Part model, mm, in its own coordinate system. A direction names the side the tool comes from. Give positions to 0.01 mm unless a question says otherwise; leave off trailing zeros. Order: outer loops, then holes, each group sorted by start corner. A loop starts at its lowest first (then second) coordinate and runs counter-clockwise, first axis right, second up. Notation, with made-up numbers: (52.25, 6.5) -> (110.25, 6.5) arc R22 cw to (110.25, 28.5) -> close; hole circle Ø8 at (61, 8). An arc over 180 degrees is marked (long way). Write item = value, one per line. Start each with the question number.
(1) Which spindle directions (+Z, -Z, +X, -X, +Y, -Y) get a long thin tool onto all of the face, cutting with end or side? Do faces 1 (the flat face through (2, 25, 3)), 2 (the flat face through (-21, 10, 3)), 3 (the flat face through (-21, 25, 3)), 4 (the flat face through (0, 0, 2)). Say none if no direction does.
(2) Saw through at C-C, the plane y = 3.5. List the corners of the cut face in (x, z), then the cut area to 3 significant figures.
(3) Saw through at A-A, the plane z = 0.75. List the corners of the cut face in (x, y).
(4) Saw through at D-D, the plane x = -20.5. List the corners of the cut face in (y, z).
(5) Probe line 1 along Y through (x, z) = (-20.5, 4.05); line 2 along Y through (x, z) = (2.5, 3.4); line 3 along Y through (x, z) = (-14, 2.55). List the from-to ranges inside material, lowest first. Write a range as from..to.
(6) Flat gauge pins, fed straight in: pin 1 (2.5 mm diameter, centred on y = 23.5, z = 1.5, fed in from -X); pin 2 (2.5 mm diameter, centred on x = -5.5, z = 3, fed in from +Y); pin 3 (1.5 mm diameter, centred on x = -13.5, z = 3, fed in from -Y); pin 4 (4 mm diameter, centred on x = 2.5, y = 31.5, fed in from +Z). Where does each tip first touch, or does it go through?
(7) Saw through at B-B, the plane x = 2.5. List the corners of the cut face in (y, z).
from build123d import *

# Parameters (mm, degrees)
SKETCH1_W           = 18
SKETCH1_H           = 35
BOSS_EXTRUDE1_DEPTH = 5
SKETCH2_W           = 5
SKETCH2_H           = 20
BOSS_EXTRUDE2_DEPTH = 5
SKETCH3_W           = 9
SKETCH3_H           = 5
BOSS_EXTRUDE3_DEPTH = 5
SKETCH4_W           = 5
SKETCH4_H           = 15
BOSS_EXTRUDE4_DEPTH = 5
SKETCH5_W           = 9
SKETCH5_H           = 5
BOSS_EXTRUDE5_DEPTH = 5
SKETCH6_R           = 2.1
CUT_EXTRUDE1_DEPTH  = 5
BOSS_EXTRUDE6_DEPTH = 5
SKETCH8_R           = 2.1
CUT_EXTRUDE2_DEPTH  = 5
BOSS_EXTRUDE7_DEPTH = 5


with BuildPart() as part:
    # Sketch1 → Boss-Extrude1 (new body)
    with BuildSketch(Plane.XY):
        with Locations((-9, 17.5)):
            Rectangle(SKETCH1_W, SKETCH1_H)
    extrude(amount=BOSS_EXTRUDE1_DEPTH)

    # Sketch2 → Boss-Extrude2 (add)
    with BuildSketch(Plane(origin=(0, 0, 0), x_dir=(0, 0, -1), z_dir=(1, 0, 0))):
        with Locations((-2.5, 15)):
            Rectangle(SKETCH2_W, SKETCH2_H)
    extrude(amount=BOSS_EXTRUDE2_DEPTH)

    # Sketch3 → Boss-Extrude3 (add)
    with BuildSketch(Plane.XZ):
        with Locations((-4.5, 2.5)):
            Rectangle(SKETCH3_W, SKETCH3_H)
    extrude(amount=BOSS_EXTRUDE3_DEPTH)

    # Sketch4 → Boss-Extrude4 (add)
    with BuildSketch(Plane.XY.offset(5)):
        with Locations((-20.5, 17.5)):
            Rectangle(SKETCH4_W, SKETCH4_H)
    extrude(amount=-BOSS_EXTRUDE4_DEPTH)

    # Sketch5 → Boss-Extrude5 (add)
    with BuildSketch(Plane(origin=(0, 35, 0), x_dir=(1, 0, 0), z_dir=(0, 1, 0))):
        with Locations((-13.5, -2.5)):
            Rectangle(SKETCH5_W, SKETCH5_H)
    extrude(amount=BOSS_EXTRUDE5_DEPTH)

    # Sketch6 → Cut-Extrude1 (cut)
    with BuildSketch(Plane(origin=(0, 0, 0), x_dir=(-1, 0, 0), z_dir=(0, 0, -1))):
        with Locations((-2.5, 15)):
            Circle(SKETCH6_R)
    extrude(amount=-CUT_EXTRUDE1_DEPTH, mode=Mode.SUBTRACT)

    # Sketch7 → Boss-Extrude6 (add)
    with BuildSketch(Plane(origin=(0, 0, 0), x_dir=(-1, 0, 0), z_dir=(0, 0, -1))):
        with BuildLine():
            Line((-5, 10.669872981), (-5, 19.330127019))
            ThreePointArc((-5, 19.330127019), (-7.5, 15), (-5, 10.669872981))
        make_face()
    extrude(amount=-BOSS_EXTRUDE6_DEPTH)

    # Sketch8 → Cut-Extrude2 (cut)
    with BuildSketch(Plane.XY.offset(5)):
        with Locations((-20.5, 17.5)):
            Circle(SKETCH8_R)
    extrude(amount=-CUT_EXTRUDE2_DEPTH, mode=Mode.SUBTRACT)

    # Sketch9 → Boss-Extrude7 (add)
    with BuildSketch(Plane.XY.offset(5)):
        with BuildLine():
            Line((-23, 13.169872981), (-23, 21.830127019))
            ThreePointArc((-23, 21.830127019), (-25.5, 17.5), (-23, 13.169872981))
        make_face()
    extrude(amount=-BOSS_EXTRUDE7_DEPTH)


solid = part.part
Results list:
q1.face_1 = +Z, -Z, +X, +Y
q1.face_2 = +Z, -Z, -X, -Y
q1.face_3 = +Z, -Z, -X, +Y
q1.face_4 = +Z, -Z, +X, -Y
q2.outline = (-18, 0) -> (0, 0) -> (0, 5) -> (-18, 5) -> close
q2.area = 90.0 mm^2
q3.outline = (-23, 10) -> (-18, 10) -> (-18, 0) -> (-9, 0) -> (-9, -5) -> (0, -5) -> (0, 5) -> (5, 5) -> (5, 10.67) arc R5 ccw to (5, 19.33) -> (5, 25) -> (0, 25) -> (0, 35) -> (-9, 35) -> (-9, 40) -> (-18, 40) -> (-18, 25) -> (-23, 25) -> (-23, 21.83) arc R5 ccw to (-23, 13.17) -> close; hole circle Ø4.2 at (-20.5, 17.5); hole circle Ø4.2 at (2.5, 15)
q4.outline = (10, 0) -> (15.4, 0) -> (15.4, 5) -> (10, 5) -> close; (19.6, 0) -> (25, 0) -> (25, 5) -> (19.6, 5) -> close
q5.line_1 = 10..15.4, 19.6..25
q5.line_2 = 5..12.9, 17.1..25
q5.line_3 = 0..40
q6.pin_1 = -23
q6.pin_2 = 35
q6.pin_3 = 0
q6.pin_4 = through
q7.outline = (5, 0) -> (12.9, 0) -> (12.9, 5) -> (5, 5) -> close; (17.1, 0) -> (25, 0) -> (25, 5) -> (17.1, 5) -> close
